Part model, mm, in its own coordinate system. A direction names the side the tool comes from. Coordinates: 2 decimals unless noted, no trailing zeros. Write each loop counter-clockwise with the first axis right and the second up, starting at its lowest first coordinate (ties: lowest second). Pieces come first, ordered by that corner, then holes. Notation, with made-up numbers: (30, 76) - (40, 76) arc R26 ccw to (40, 101) - close; hole circle Ø2 at (-16, 63). An arc over 180 degrees is marked (long way). Write each question's results on one line, items separated by ' | '.
Autodesk Inventor part; units mm, degrees
ref_plane "YZ Plane" through (0, 0, 0) normal (1, 0, 0) x (0, 1, 0)
ref_plane "XZ Plane" through (0, 0, 0) normal (0, 1, 0) x (-1, 0, 0)
ref_plane "XY Plane" through (0, 0, 0) normal (0, 0, 1) x (1, 0, 0)
sketch "Sketch1" plane through (0, 0, 0) normal (0, 1, 0) x (-1, 0, 0)
  line L0 (125.7746, -116.0471) -> (66.7746, -116.0471)
  line L1 (66.7746, -116.0471) -> (66.7746, 37.4129)
  line L2 (66.7746, 37.4129) -> (125.7746, 37.4129)
  line L3 (125.7746, 37.4129) -> (125.7746, -116.0471)
  point P0 (0, 0)
  dimension "d0" = 59
  dimension "d1" = 153.46
extrude "Extrusion1" add sketch "Sketch1" along normal blind 49
sketch "Sketch2" plane through (0, 0, 0) normal (0, -1, 0) x (1, 0, 0)
  line L0 (-125.7746, 37.4129) -> (-66.7746, 37.4129)
  line L1 (-66.7746, -116.0471) -> (-125.7746, -116.0471)
  line L2 (-85.8246, 37.4129) -> (-106.7246, 37.4129)
  line L3 (-106.7246, 37.4129) -> (-106.7246, -116.0471)
  line L4 (-106.7246, -116.0471) -> (-85.8246, -116.0471)
  line L5 (-85.8246, -116.0471) -> (-85.8246, 37.4129)
  line L6 (-66.7746, 37.4129) -> (-66.7746, -116.0471)
  line L7 (-125.7746, -116.0471) -> (-125.7746, 37.4129)
  point P0 (0, 0)
  dimension "d4" = 19.05
  dimension "d5" = 19.05
extrude "Extrusion2" add sketch "Sketch2" along normal blind 3.22 contours L0 L5 L1 L3
sketch "Sketch3" plane through (0, 49, 0) normal (0, 1, 0) x (1, 0, 0)
  line L0 (-125.7746, -37.4129) -> (-66.7746, -37.4129)
  line L1 (-106.7246, 116.0471) -> (-125.7746, 116.0471)
  line L2 (-85.8246, -37.4129) -> (-106.7246, -37.4129)
  line L3 (-106.7246, -37.4129) -> (-106.7246, 116.0471)
  line L4 (-106.7246, 116.0471) -> (-85.8246, 116.0471)
  line L5 (-85.8246, 116.0471) -> (-85.8246, -37.4129)
  line L6 (-66.7746, -37.4129) -> (-66.7746, 116.0471)
  line L7 (-125.7746, 116.0471) -> (-125.7746, -37.4129)
  point P0 (0, 0)
  dimension "d8" = 19.05
  dimension "d9" = 19.05
extrude "Extrusion3" add sketch "Sketch3" along normal blind 5 contours L3 L4 L5 L0
sketch "Sketch4" plane through (-66.7746, 0, 37.4129) normal (1, 0, 0) x (0, 0, -1)
  line L0 (0, 0) -> (0, 49)
  line L1 (153.46, 0) -> (153.46, 49)
  line L2 (0, 36.3) -> (153.46, 36.3)
  line L3 (153.46, 36.3) -> (153.46, 12.7)
  line L4 (153.46, 12.7) -> (0, 12.7)
  line L5 (0, 12.7) -> (0, 36.3)
  line L6 (0, 49) -> (153.46, 49)
  line L7 (0, 0) -> (153.46, 0)
  point P0 (37.4129, 0)
  point P1 (0, 12.7)
  dimension "d12" = 12.7
  dimension "d13" = 12.7
extrude "Extrusion4" add sketch "Sketch4" along normal blind 4 contours L0 L2 L1 L4
sketch "Sketch5" plane through (-125.7746, 0, -116.0471) normal (-1, 0, 0) x (0, 0, 1)
  line L0 (153.46, 0) -> (153.46, 49)
  line L1 (0, 0) -> (0, 49)
  line L2 (153.46, 12.7) -> (0, 12.7)
  line L3 (0, 12.7) -> (0, 36.3)
  line L4 (0, 36.3) -> (153.46, 36.3)
  line L5 (153.46, 36.3) -> (153.46, 12.7)
  line L6 (0, 0) -> (153.46, 0)
  line L7 (0, 49) -> (153.46, 49)
  point P0 (116.0471, 0)
  point P1 (0, 12.7)
  dimension "d16" = 12.7
  dimension "d17" = 12.7
extrude "Extrusion5" add sketch "Sketch5" along normal blind 4 contours L2 L1 L4 L0
sketch "Sketch6" plane through (-66.7746, 0, -116.0471) normal (0, 0, -1) x (-1, 0, 0)
  line L0 (63, -3.22) -> (-4, -3.22)
  line L1 (-4, -3.22) -> (-4, 54)
  line L2 (-4, 54) -> (63, 54)
  line L3 (63, 54) -> (63, -3.22)
  line L4 (19.05, 54) -> (39.95, 54)
  line L5 (63, 36.3) -> (63, 12.7)
  line L6 (-4, 12.7) -> (-4, 36.3)
  point P0 (-66.7746, 0)
  dimension "d20" = 0
  dimension "d21" = 0
  dimension "d22" = 0
extrude "Extrusion6" add sketch "Sketch6" along normal blind 6.395
sketch "Sketch7" plane through (-129.7746, 0, -116.0471) normal (-1, 0, 0) x (0, 0, 1)
  line L0 (153.46, 54) -> (0, 54)
  line L1 (153.46, -3.22) -> (0, -3.22)
  line L2 (38.1, 54) -> (63.5, 54)
  line L3 (63.5, 54) -> (63.5, -3.22)
  line L4 (63.5, -3.22) -> (38.1, -3.22)
  line L5 (38.1, -3.22) -> (38.1, 54)
  line L6 (101.6, 54) -> (127, 54)
  line L7 (127, 54) -> (127, -3.22)
  line L8 (127, -3.22) -> (101.6, -3.22)
  line L9 (101.6, -3.22) -> (101.6, 54)
  line L10 (0, 36.3) -> (0, 54)
  point P0 (116.0471, 0)
  point P1 (127, -3.22)
  dimension "d25" = 38.1
  dimension "d26" = 38.1
  dimension "d27" = 25.4
  dimension "d28" = 25.4
extrude "Extrusion7" add sketch "Sketch7" against normal up to surface (67 mm away) contours L7 L1 L9 L0 | L3 L1 L5 L0
sketch "Sketch8" plane through (-125.7746, 0, 37.4129) normal (0, 0, 1) x (1, 0, 0)
  line L0 (39.95, 49) -> (59, 49)
  line L1 (-4, 54) -> (19.05, 54)
  line L2 (42.2021, 49) -> (16.8021, 49)
  line L3 (16.8021, 49) -> (16.8021, 54)
  line L4 (16.8021, 54) -> (42.2021, 54)
  line L5 (42.2021, 54) -> (42.2021, 49)
  line L6 (19.05, 49) -> (19.05, 54)
  line L7 (0, 0) -> (19.05, 0)
  line L8 (39.95, -3.22) -> (63, -3.22)
  line L9 (16.8021, 0) -> (42.2021, 0)
  line L10 (42.2021, 0) -> (42.2021, -3.22)
  line L11 (42.2021, -3.22) -> (16.8021, -3.22)
  line L12 (16.8021, -3.22) -> (16.8021, 0)
  point P0 (125.7746, 0)
  point P1 (42.2021, 51.5)
  point P2 (16.8021, 51.5)
  point P3 (19.05, 51.5)
  dimension "d31" = 25.4
  dimension "d32" = 2.2479
extrude "Extrusion8" add sketch "Sketch8" along normal blind 6.35
sketch "Sketch9" plane through (0, 54, 0) normal (0, 1, 0) x (1, 0, 0)
  line L0 (-118.2456, -83.2824) -> (-137.2956, -83.2824)
  line L1 (-137.2956, -83.2824) -> (-137.2956, -80.1074)
  line L2 (-137.2956, -80.1074) -> (-118.2456, -80.1074)
  line L3 (-118.2456, -80.1074) -> (-118.2456, -83.2824)
  line L4 (-86.7475, -39.0639) -> (-105.7975, -39.0639)
  line L5 (-105.7975, -39.0639) -> (-105.7975, -42.2389)
  line L6 (-105.7975, -42.2389) -> (-86.7475, -42.2389)
  line L7 (-86.7475, -42.2389) -> (-86.7475, -39.0639)
  line L8 (-83.5725, -43.7629) -> (-108.9725, -43.7629)
  line L9 (-83.5725, -37.4129) -> (-83.5725, -43.7629)
  point P0 (0, 0)
  point P1 (-118.2456, -81.6949)
  point P2 (-137.2956, -81.6949)
  point P3 (-105.7975, -40.6514)
  point P4 (-86.7475, -40.6514)
  point P5 (-83.5725, -40.5879)
  dimension "d35" = 3.175
  dimension "d36" = 19.05
  dimension "d37" = 19.05
  dimension "d38" = 3.175
  dimension "d39" = 1.524
  dimension "d40" = 3.175
extrude "Extrusion9" cut sketch "Sketch9" against normal up to surface (57.22 mm away) contours L7 L6 L5 L4
sketch "Sketch10" plane through (-66.7746, 12.7, 37.4129) normal (0, 0, 1) x (1, 0, 0)
  line L0 (-59, 23.6) -> (-59, 36.3)
  line L1 (0, 0) -> (0, -12.7)
  line L2 (-59, 36.3) -> (0, 36.3)
  line L3 (0, 36.3) -> (0, -12.7)
  line L4 (0, -12.7) -> (-59, -12.7)
  line L5 (-59, -12.7) -> (-59, 36.3)
  point P0 (66.7746, -12.7)
  point P1 (-59, 23.6)
extrude "Extrusion10" cut sketch "Sketch10" against normal up to surface (153.46 mm away)
sketch "Sketch11" plane through (0, 54, 0) normal (0, 1, 0) x (1, 0, 0)
  line L0 (-85.8246, 116.0471) -> (-85.8246, 77.9471)
  line L1 (-129.7746, 52.5471) -> (-106.7246, 52.5471)
  line L2 (-85.8246, 52.5471) -> (-85.8246, 14.4471)
  line L3 (-129.7746, -10.9529) -> (-106.7246, -10.9529)
  circle A0 centre (-96.2746, 65.2471) radius 1.35
  circle A1 centre (-96.2746, 1.7471) radius 1.35
  point P0 (0, 0)
  dimension "d45" = 2.7
  dimension "d46" = 2.7
  dimension "d47" = 63.5
extrude "Extrusion11" cut sketch "Sketch11" against normal up to surface (57.22 mm away)
sketch "Sketch12" plane through (-108.9725, 49, 43.7629) normal (0, -1, 0) x (1, 0, 0)
  circle A0 centre (12.6979, -45.51) radius 1.35
  circle A1 centre (12.6979, -45.51) radius 3.175
  circle A2 centre (12.6979, -109.01) radius 1.35
  circle A3 centre (12.6979, -109.01) radius 3.175
  point P0 (108.9725, -43.7629)
  dimension "d50" = 6.35
  dimension "d51" = 6.35
extrude "Extrusion12" cut sketch "Sketch12" against normal blind 2 contours A0 | A1 | A2 | A3
sketch "Sketch13" plane through (-129.7746, 0, -116.0471) normal (-1, 0, 0) x (0, 0, 1)
  line L0 (153.46, 36.3) -> (127, 36.3)
  line L1 (127, 12.7) -> (153.46, 12.7)
  line L2 (153.46, 36.3) -> (146.2804, 36.3)
  line L3 (146.2804, 36.3) -> (146.2804, 12.7)
  line L4 (146.2804, 12.7) -> (153.46, 12.7)
  line L5 (153.46, 12.7) -> (153.46, 36.3)
  point P0 (116.0471, 0)
extrude "Extrusion13" cut sketch "Sketch13" against normal up to surface (67 mm away)
sketch "Sketch14" plane through (-66.7746, 0, -122.4421) normal (0, 0, -1) x (-1, 0, 0)
  line L0 (-4, 36.3) -> (-4, 54)
  line L1 (-4, 54) -> (19.05, 54)
  line L2 (19.05, 54) -> (19.05, 36.3)
  line L3 (19.05, 36.3) -> (-4, 36.3)
  line L4 (-4, 36.3) -> (-4, 54)
  line L5 (63, -3.22) -> (63, 54)
  line L6 (63, 54) -> (40.73, 54)
  line L7 (40.73, 54) -> (40.73, 36.3)
  line L8 (40.73, 36.3) -> (63, 36.3)
  line L9 (63, 36.3) -> (63, 54)
  line L10 (63, 12.7) -> (63, -3.22)
  line L11 (63, -3.22) -> (39.95, -3.22)
  line L12 (63, 12.7) -> (39.95, 12.7)
  line L13 (39.95, 12.7) -> (39.95, -3.22)
  line L14 (39.95, -3.22) -> (63, -3.22)
  line L15 (63, -3.22) -> (63, 12.7)
  line L16 (-4, 12.7) -> (-4, -3.22)
  line L17 (-4, -3.22) -> (19.05, -3.22)
  line L18 (19.05, -3.22) -> (19.05, 12.7)
  line L19 (19.05, 12.7) -> (-4, 12.7)
  line L20 (-4, 12.7) -> (-4, -3.22)
  point P0 (-66.7746, 0)
  point P1 (19.05, 54)
  point P2 (-4, 12.7)
  point P3 (63, 36.3)
  point P4 (63, 36.3)
  dimension "d56" = 0
  dimension "d59" = 0
  dimension "d60" = 0
extrude "Extrusion14" cut sketch "Sketch14" against normal up to surface (6.395 mm away)
properties part number "battery holder v2"
(1) Flat gauge pins, fed straight in: P1, Ø5.5, axis at y = 48.5, z = -97.5, coming from the +X side; P2, Ø2.5, axis at x = -85, y = -1, coming from the -Z side; P3, Ø5, axis at x = -115, y = 26.5, coming from the +Z side; P4, Ø18, axis at x = -119.5, z = -99, coming from the +Y side. Where does each tip first touch, or does it go through?
Return value:
P1: stops at x = -85.82 | P2: stops at z = -122.44 | P3: stops at z = -116.05 | P4: stops at y = 36.3
(2) Two-plate mould, pull along Y, no slides. Class faces 6 (the flat face through (-125.775, 24, -42)), 7 (the flat face through (-65, 12.7, 20)), 8 (the flat face through (-72, 50, -77.947)): released by +Y, released by -Y, zero draft, split by the parting line, or undercut.
Return value:
face 6: undercut | face 7: released by -Y | face 8: zero draft
(3) Wall check: line 1 (Y direction, x = -97.5, z = -61.5); line 2 (X direction, y = 16.5, z = -87); line 3 (Z direction, x = -100, y = 21.5). Give the ranges that are in metal, low to high. Write a range as from..to.
Return value:
line 1: y = -3.22..0, 49..54 | line 2: x = -129.77..-125.77, -66.77..-62.77 | line 3: z = -122.44..-116.05
(4) 3-axis set-ups, long thin cutter, end or side, ignore diameter. For faces 1 (the flat face through (-72, 50, -14.447)), 2 (the flat face through (-106.725, -2, -33)), 3 (the flat face through (-85.825, -1, -109)), 4 (the flat face through (-124, -1, -14.447)), 5 (the flat face through (-121, 49.2, -52.547)): which of +Z, -Z, +X, -X, +Y, -Y reach the whole face in a straight line?
Return value:
face 1: +X, +Y | face 2: -X, +Y, -Y | face 3: -Z, +X, -Y | face 4: -X, -Y | face 5: -X, +Y
(5) Saw through at D-D on z = -81.5. Write the cut outline in (x, y), then the cut area to 3 significant figures.
Return value:
outline: (-129.77, 12.7) - (-125.77, 12.7) - (-125.77, 36.3) - (-129.77, 36.3) - close; (-106.72, -3.22) - (-85.82, -3.22) - (-85.82, 0) - (-106.72, 0) - close; (-106.72, 49) - (-85.82, 49) - (-85.82, 54) - (-106.72, 54) - close; (-66.77, 12.7) - (-62.77, 12.7) - (-62.77, 36.3) - (-66.77, 36.3) - close | area: 361 mm^2
(6) Saw through at C-C on x = -90. Write the cut outline in (y, z), then the cut area to 3 significant figures.
Return value:
outline: (-3.22, -122.44) - (54, -122.44) - (54, 39.06) - (49, 39.06) - (49, -116.05) - (0, -116.05) - (0, 39.06) - (-3.22, 39.06) - close; (-3.22, 42.24) - (0, 42.24) - (0, 43.76) - (-3.22, 43.76) - close; (49, 42.24) - (54, 42.24) - (54, 43.76) - (49, 43.76) - close | area: 1,650 mm^2
(7) Saw through at A-A on x = -115. Write the cut outline in (y, z), then the cut area to 3 significant figures.
Return value:
outline: (-3.22, -77.95) - (0, -77.95) - (0, -52.55) - (-3.22, -52.55) - close; (-3.22, -14.45) - (0, -14.45) - (0, 10.95) - (-3.22, 10.95) - close; (12.7, -122.44) - (36.3, -122.44) - (36.3, -116.05) - (12.7, -116.05) - close; (49, -77.95) - (54, -77.95) - (54, -52.55) - (49, -52.55) - close; (49, -14.45) - (54, -14.45) - (54, 10.95) - (49, 10.95) - close | area: 568 mm^2
(8) Saw through at B-B on y = 46. Write the cut outline in (x, z), then the cut area to 3 significant figures.
Return value:
outline: (-129.77, -77.95) - (-125.77, -77.95) - (-125.77, -52.55) - (-129.77, -52.55) - close; (-129.77, -14.45) - (-125.77, -14.45) - (-125.77, 10.95) - (-129.77, 10.95) - close; (-107.5, -122.44) - (-85.82, -122.44) - (-85.82, -116.05) - (-107.5, -116.05) - close; (-66.77, -77.95) - (-62.77, -77.95) - (-62.77, -52.55) - (-66.77, -52.55) - close; (-66.77, -14.45) - (-62.77, -14.45) - (-62.77, 10.95) - (-66.77, 10.95) - close | area: 545 mm^2
